Can you work these out from the model? Positions are in its coordinate system, mm. Face numbers are marked on the shaded views. A direction names the side the tool comes from. Give positions to 0.01 mm unless a question says otherwise; leave off trailing zeros. Order: outer loops, then holes, each group sorted by start corner. A loop starts at its lowest first (then second) coordinate and runs counter-clockwise, first axis right, second up. Notation, with made-up numbers: (30, 54.5) - (70, 54.5) arc R22 ccw to (70, 89.5) - close; hole circle Ø7 at (-33.5, 51.5). An arc over 180 degrees is marked (long way). Use one line per item in the form item = value. Start each with the question number.
1) Which directions (+Z, -Z, +X, -X, +Y, -Y) give clear straight access to the entire face, cutting with the end or side of a thin tool? Please do the marked faces 5, 6 and 7.
2) Please list where these lines run through material, in increasing order: probe 1 along Y at (x, z) = (-11.5, 1.75); probe 2 along Y at (x, z) = (0, 12.25); probe 3 along X at (y, z) = (-1.25, 4.75).
3) We'd pull the mould along Z, two halves only. Please class the marked faces 1, 2, 3 and 4: released by +Z, released by -Z, zero draft, split by the parting line, or undercut.
4) Suppose I cut it at D-D, the plane z = 4.5. Write out the boundary of the cut face in (x, y).
5) For pin 1 (3.5 mm diameter, centred on x = 0, y = 0, fed in from -Z); pin 2 (5 mm diameter, centred on x = -9.5, z = 16.5, fed in from +Y); pin 3 (1.5 mm diameter, centred on x = -1.5, z = 15.5, fed in from -Y); pin 4 (13 mm diameter, centred on x = -9.5, z = 8.5, fed in from -Y), each with a flat end and sliding along its axis, tell me the tip position at first contact or that it passes through.
6) Suppose I cut it at A-A, the plane z = 12.5. State how many separate pieces and enclosed holes the cut face has, and give its area (3 significant figures).
7) Suppose I cut it at B-B, the plane x = 0. Write out the boundary of the cut face in (y, z), and give its area (3 significant figures).
8) Suppose I cut it at C-C, the plane y = -3.5. Write out the boundary of the cut face in (x, z), and give its area (3 significant figures).
```python
from build123d import *

# Parameters (mm, degrees)
F1_DEPTH = 25
F2_R     = 1.6
F3_DEPTH = 10.001
F2_R_2   = 3
F4_DEPTH = 1.5
F5_R     = 2
F6_R     = 1.6
F7_DEPTH = 7.501
F8_DEPTH = 1.5
F9_R     = 2


with BuildPart() as f1:
    # F0 (on Top) → F1 (new body)
    with BuildSketch(Plane.XY):
        with BuildLine():
            ThreePointArc((-2.828427, 1), (3, 0), (-2.828427, -1))
            Line((-2.828427, -1), (-14.472136, -1))
            Line((-14.472136, -1), (-14.472136, -4))
            Line((-14.472136, -4), (-4.472136, -4))
            ThreePointArc((-4.472136, -4), (1.41761, -5.830127), (5.809475, -1.5))
            Line((5.809475, -1.5), (15.809475, -1.5))
            Line((15.809475, -1.5), (15.809475, 1.5))
            Line((15.809475, 1.5), (5.809475, 1.5))
            ThreePointArc((5.809475, 1.5), (1.41761, 5.830127), (-4.472136, 4))
            Line((-4.472136, 4), (-14.472136, 4))
            Line((-14.472136, 4), (-14.472136, 1))
            Line((-14.472136, 1), (-2.828427, 1))
        make_face()
    extrude(amount=F1_DEPTH)

    # F2 (on face) → F3 (cut, through all)
    with BuildSketch(Plane(origin=(0, 4, 0), x_dir=(-1, 0, 0), z_dir=(0, 1, 0))):
        with Locations((9.472136, 12.5)):
            Circle(F2_R)
    extrude(amount=-F3_DEPTH, mode=Mode.SUBTRACT)

    # F2 (on face) → F4 (cut)
    with BuildSketch(Plane(origin=(0, 4, 0), x_dir=(-1, 0, 0), z_dir=(0, 1, 0))):
        with Locations((9.472136, 12.5)):
            Circle(F2_R_2)
        with Locations((9.472136, 12.5)):
            Circle(F2_R, mode=Mode.SUBTRACT)
    extrude(amount=-F4_DEPTH, mode=Mode.SUBTRACT)

    # F5
    f5_edges = [f1.edges().sort_by_distance(p)[0] for p in [
        (-14.472136, 2.5, 0),
        (-14.472136, -2.5, 0),
        (-14.472136, -2.5, 25),
        (-14.472136, 2.5, 25),
    ]]
    fillet(f5_edges, radius=F5_R)

    # F6 (on face) → F7 (cut, through all)
    with BuildSketch(Plane(origin=(0, 1.5, 0), x_dir=(-1, 0, 0), z_dir=(0, 1, 0))):
        with Locations((-10.809475, 12.5)):
            Circle(F6_R)
    extrude(amount=-F7_DEPTH, mode=Mode.SUBTRACT)

    # F6 (on face) → F8 (cut)
    with BuildSketch(Plane(origin=(0, 1.5, 0), x_dir=(-1, 0, 0), z_dir=(0, 1, 0))):
        Polygon((-13.809475, 14.232051), (-13.809475, 10.767949), (-10.809475, 9.035898), (-7.809475, 10.767949), (-7.809475, 14.232051), (-10.809475, 15.964102), align=None)
        with Locations((-10.809475, 12.5)):
            Circle(F6_R, mode=Mode.SUBTRACT)
    extrude(amount=-F8_DEPTH, mode=Mode.SUBTRACT)

    # F9
    f9_edges = [f1.edges().sort_by_distance(p)[0] for p in [
        (15.809475, 0, 25),
        (15.809475, 0, 0),
    ]]
    fillet(f9_edges, radius=F9_R)


solid = f1.part
```
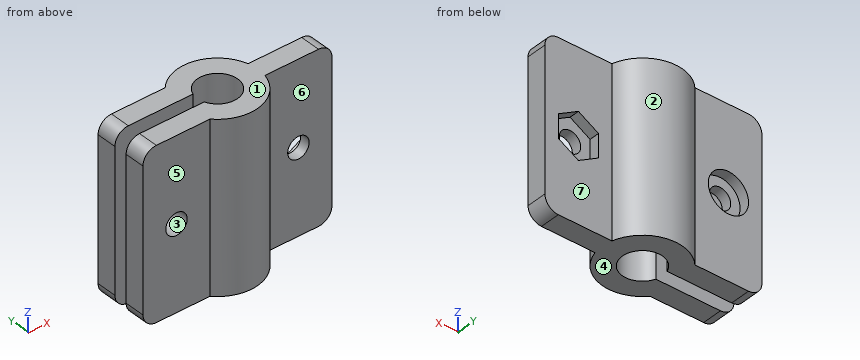
Result sheet:
q1.face_5 = +Z, -Z, -X, -Y
q1.face_6 = +Z, -Z, +X, -Y
q1.face_7 = +Z, -Z, +X, +Y
q2.probe_1 = -4 to -1, 1 to 4
q2.probe_2 = -6 to -3, 3 to 6
q2.probe_3 = -14.47 to -2.73, 2.73 to 15.81
q3.face_1 = released by +Z
q3.face_2 = zero draft
q3.face_3 = undercut
q3.face_4 = released by -Z
q4.outline = (-14.47, -4) - (-4.47, -4) arc R6 ccw to (5.81, -1.5) - (15.81, -1.5) - (15.81, 1.5) - (5.81, 1.5) arc R6 ccw to (-4.47, 4) - (-14.47, 4) - (-14.47, 1) - (-2.83, 1) arc R3 cw (long way) to (-2.83, -1) - (-14.47, -1) - close
q5.pin_1 = through
q5.pin_2 = 4
q5.pin_3 = -5.95
q5.pin_4 = -5.2
q6.separate_pieces = 4
q6.enclosed_holes = 0
q6.area = 126 mm²
q7.outline = (-6, 0) - (-3, 0) - (-3, 25) - (-6, 25) - close; (3, 0) - (6, 0) - (6, 25) - (3, 25) - close
q7.area = 150 mm²
q8.outline = (-14.47, 2) arc R2 ccw to (-12.47, 0) - (4.87, 0) - (4.87, 25) - (-12.47, 25) arc R2 ccw to (-14.47, 23) - close; hole circle Ø3.2 at (-9.47, 12.5)
q8.area = 474 mm²
